Design review of the part built by this model. Coordinates are the model's own, in mm. Face numbers are marked on the shaded views. Coordinates: 2 decimals unless noted, no trailing zeros. Write each loop counter-clockwise with the first axis right and the second up, starting at its lowest first coordinate (ties: lowest second). Pieces come first, ordered by that corner, then holes. Notation, with made-up numbers: (-38, 41) -> (-29, 41) arc R30 ccw to (-29, 80) -> close; hole circle Ø8 at (78.25, 76). An arc over 180 degrees is marked (long way). Return JSON: item names as keys, results as strings. Group by question number.
from build123d import *

# Parameters (mm, degrees)
F1_DEPTH = 25.4


# Not quite as in the source:
# - ends of sketch curves that miss each other by under 0.0002 mm in the source are joined


with BuildPart() as f1:
    # F0 (on Front) → F1 (new body)
    with BuildSketch(Plane.XZ):
        with BuildLine():
            ThreePointArc((7.9345325801, 55.8050164826), (5.535399088, 50.3331676174), (0, 48.0845394904))
            ThreePointArc((0, 48.0845394904), (-5.53484385, 50.3326274112), (-7.9344900677, 55.8034677281))
            ThreePointArc((-7.9344900677, 55.8034677281), (-20.6052011609, 52.4624086595), (-32.1621766165, 46.2861708383))
            ThreePointArc((-32.1621766165, 46.2861708383), (-30.8592654267, 43.9476457313), (-30.4078463876, 41.3089911317))
            ThreePointArc((-30.4078463876, 41.3089911317), (-31.0665806395, 38.1430038554), (-32.9334464969, 35.5025080461))
            ThreePointArc((-32.9334464969, 35.5025080461), (-38.3527879746, 33.37149462), (-43.7681241803, 35.5126658077))
            ThreePointArc((-43.7681241803, 35.5126658077), (-51.6631141521, 22.5336801806), (-55.8055284532, 7.9177526246))
            ThreePointArc((-55.8055284532, 7.9177526246), (-50.5579583584, 5.4112130729), (-48.4275815127, 0))
            ThreePointArc((-48.4275815127, 0), (-50.5584477046, -5.4117381745), (-55.8069604277, -7.917853693))
            ThreePointArc((-55.8069604277, -7.917853693), (-51.6665413057, -22.5360169357), (-43.772503534, -35.5174627239))
            ThreePointArc((-43.772503534, -35.5174627239), (-38.3573927277, -33.3769597298), (-32.9385406353, -35.5079735997))
            ThreePointArc((-32.9385406353, -35.5079735997), (-31.0716747779, -38.1484694089), (-30.412940526, -41.3144566852))
            ThreePointArc((-30.412940526, -41.3144566852), (-30.8645222652, -43.9535728332), (-32.1678845367, -46.2923987991))
            ThreePointArc((-32.1678845367, -46.2923987991), (-20.6005666804, -52.4744238707), (-7.9177489459, -55.8160418449))
            ThreePointArc((-7.9177489459, -55.8160418449), (0.0007699496, -48.4381469932), (7.917857362, -55.8175779229))
            ThreePointArc((7.917857362, -55.8175779229), (20.6543242596, -52.4575865986), (32.263311311, -46.2335565237))
            ThreePointArc((32.263311311, -46.2335565237), (31.0776824279, -40.9625014731), (33.540338967, -36.1536492228))
            ThreePointArc((33.540338967, -36.1536492228), (38.5262504819, -34.0340714863), (43.7106191867, -35.607044642))
            ThreePointArc((43.7106191867, -35.607044642), (51.6543788303, -22.5889167608), (55.8178964863, -7.917853693))
            ThreePointArc((55.8178964863, -7.917853693), (48.4385176038, -0.0007177684), (55.8164645119, 7.9177526246))
            ThreePointArc((55.8164645119, 7.9177526246), (51.6724507462, 22.537346487), (43.7740191713, 35.5188777315))
            ThreePointArc((43.7740191713, 35.5188777315), (38.4803716898, 33.3779972711), (33.1194704023, 35.3444179256))
            ThreePointArc((33.1194704023, 35.3444179256), (33.0283665185, 35.4254890622), (32.9385189369, 35.5079503192))
            ThreePointArc((32.9385189369, 35.5079503192), (30.4331832399, 40.7476116526), (32.166542765, 46.2907355552))
            ThreePointArc((32.166542765, 46.2907355552), (20.6072932493, 52.4658819521), (7.9345325801, 55.8050164826))
        make_face()
        with BuildLine():
            ThreePointArc((0, 38.1), (13.962710806, 35.4492976933), (25.9825875048, 27.8660213621))
            ThreePointArc((25.9825875048, 27.8660213621), (34.9475216227, 15.1899725896), (38.1109370587, -0.010193824))
            ThreePointArc((38.1109370587, -0.010193824), (15.1973926464, -34.9527404783), (-25.9825835021, -27.8660170726))
            ThreePointArc((-25.9825835021, -27.8660170726), (-38.1, 0), (-25.9825875048, 27.8660213621))
            ThreePointArc((-25.9825875048, 27.8660213621), (-13.962710806, 35.4492976933), (0, 38.1))
        make_face(mode=Mode.SUBTRACT)
        with BuildLine():
            ThreePointArc((-32.1621766165, 46.2861708383), (-20.6052011609, 52.4624086595), (-7.9344900677, 55.8034677281))
            ThreePointArc((-7.9344900677, 55.8034677281), (-5.6894120792, 61.5568833403), (0, 63.9595394904))
            Line((0, 63.9595394904), (0, 73.9440789808))
            ThreePointArc((0, 73.9440789808), (-27.1479472531, 68.9440014522), (-50.7331165271, 54.5999571944))
            Line((-50.7331165271, 54.5999571944), (-43.7572462783, 47.1154742172))
            ThreePointArc((-43.7572462783, 47.1154742172), (-37.7790864379, 49.2262669207), (-32.1621766165, 46.2861708383))
        make_face()
        with BuildLine():
            ThreePointArc((7.9375, 56.0220394904), (7.9367581103, 55.9135178434), (7.9345325801, 55.8050164826))
            ThreePointArc((7.9345325801, 55.8050164826), (20.6072932493, 52.4658819521), (32.166542765, 46.2907355552))
            ThreePointArc((32.166542765, 46.2907355552), (37.7835970754, 49.2316689925), (43.7623187183, 47.1209164903))
            Line((43.7623187183, 47.1209164903), (50.7331165271, 54.5999571944))
            ThreePointArc((50.7331165271, 54.5999571944), (27.1479472531, 68.9440014522), (0, 73.9440789808))
            Line((0, 73.9440789808), (0, 63.9595394904))
            ThreePointArc((0, 63.9595394904), (5.6126600757, 61.634699566), (7.9375, 56.0220394904))
        make_face()
        with BuildLine():
            ThreePointArc((-43.7681241803, 35.5126658077), (-46.2828428993, 41.3164327187), (-43.7572462783, 47.1154742172))
            Line((-43.7572462783, 47.1154742172), (-50.7331165271, 54.5999571944))
            ThreePointArc((-50.7331165271, 54.5999571944), (-31.1494504015, -71.7983666167), (76.2, -2.2559210192))
            ThreePointArc((76.2, -2.2559210192), (69.5922116943, 28.7821857449), (50.9148537664, 54.4372678657))
            Line((50.9148537664, 54.4372678657), (43.9381604406, 46.9519018008))
            ThreePointArc((43.9381604406, 46.9519018008), (45.6769666267, 44.3682185312), (46.2879188276, 41.3144334048))
            ThreePointArc((46.2879188276, 41.3144334048), (45.6323737155, 38.1557882425), (43.7740191713, 35.5188777315))
            ThreePointArc((43.7740191713, 35.5188777315), (51.6724507462, 22.537346487), (55.8164645119, 7.9177526246))
            ThreePointArc((55.8164645119, 7.9177526246), (61.7872306442, 5.8071231544), (64.3135175714, 0))
            ThreePointArc((64.3135175714, 0), (61.7877557458, -5.8066338081), (55.8178964863, -7.917853693))
            ThreePointArc((55.8178964863, -7.917853693), (51.6543788303, -22.5889167608), (43.7106191867, -35.607044642))
            ThreePointArc((43.7106191867, -35.607044642), (46.0506031098, -38.4080721744), (46.8897388577, -41.9601323083))
            ThreePointArc((46.8897388577, -41.9601323083), (46.2310046059, -45.1261195846), (44.3641387485, -47.7666153939))
            ThreePointArc((44.3641387485, -47.7666153939), (37.9546080225, -49.8346887381), (32.263311311, -46.2335565237))
            ThreePointArc((32.263311311, -46.2335565237), (20.6543242596, -52.4575865986), (7.917857362, -55.8175779229))
            ThreePointArc((7.917857362, -55.8175779229), (7.9325878205, -56.0964396499), (7.9375, -56.3756469558))
            ThreePointArc((7.9375, -56.3756469558), (-0.2799767777, -64.3082076555), (-7.9177489459, -55.8160418449))
            ThreePointArc((-7.9177489459, -55.8160418449), (-20.6005666804, -52.4744238707), (-32.1678845367, -46.2923987991))
            ThreePointArc((-32.1678845367, -46.2923987991), (-37.784668716, -49.2317673719), (-43.7623404168, -47.1209397708))
            ThreePointArc((-43.7623404168, -47.1209397708), (-46.2879374814, -41.3214088869), (-43.772503534, -35.5174627239))
            ThreePointArc((-43.772503534, -35.5174627239), (-51.6665413057, -22.5360169357), (-55.8069604277, -7.917853693))
            ThreePointArc((-55.8069604277, -7.917853693), (-64.3025814803, 0.0007177684), (-55.8055284532, 7.9177526246))
            ThreePointArc((-55.8055284532, 7.9177526246), (-51.6631141521, 22.5336801806), (-43.7681241803, 35.5126658077))
        make_face()
    extrude(amount=F1_DEPTH)


solid = f1.part
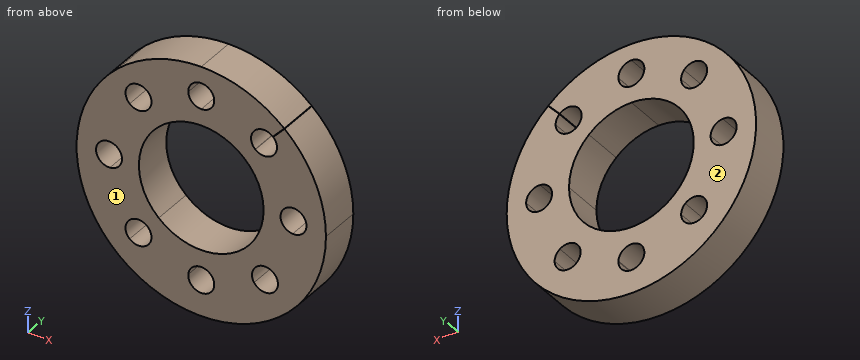
Q1. For P1, Ø1, axis at x = 7.5, y = -11.5, coming from the +Z side; P2, Ø5, axis at x = -29, z = 52, coming from the +Y side; P3, Ø1.5, axis at y = -5.5, z = 36, coming from the +X side; P4, Ø12, axis at x = 16.5, y = -11, coming from the -Z side, all flat-tipped, find the tip position at first contact; note any pin that passes through.
Q2. We need section A-A on x = -22.5. Write out the cut boundary in (y, z), plus the area to 3 significant figures.
Q3. We need section C-C on y = -9.25. State how many separate pieces and enclosed holes the cut face has, plus the area to 3 significant figures.
Q4. The part is to be moulded in two halves that separate along Y. For the marked faces 1 and 2, say which applies: +Y half, -Y half, draft (parallel to the pull), parting line (faces both ways), or undercut.
Q5. Wall thickness on L1, parallel to Z at x = -0.5, y = -7; L2, parallel to Z at x = -45, y = -19; L3, parallel to X at y = -19.5, z = 53: over which ranges is each line inside the solid? List them lowest first.
Q6. We need section B-B on x = 41. Write out the cut boundary in (y, z).
Q7. We need section D-D on x = -5.5. Write out the cut boundary in (y, z), plus the area to 3 significant figures.
Findings below:
{
 "1": {"P1": "stops at z = 73.62", "P2": "stops at y = 0", "P3": "stops at x = 66.33", "P4": "stops at z = -77.73"},
 "2": {"outline": "(-25.4, -75.06) -> (0, -75.06) -> (0, -30.75) -> (-25.4, -30.75) -> close; (-25.4, 30.75) -> (0, 30.75) -> (0, 70.55) -> (-25.4, 70.55) -> close", "area": "2,140 mm^2"},
 "3": {"separate pieces": "1", "enclosed holes": "8", "area": "12,100 mm^2"},
 "4": {"face 1": "-Y half", "face 2": "+Y half"},
 "5": {"L1": "z = -78.45 to -64.3, -48.45 to -38.11, 38.1 to 48.1, 63.94 to 73.94", "L2": "z = -63.75 to -45.65, -36.98 to 36.98, 45.64 to 59.24", "L3": "x = -52.47 to -7.34, 7.34 to 49.24, 49.58 to 52.47"},
 "6": {"outline": "(-25.4, -66.49) -> (0, -66.49) -> (0, -49.63) -> (-25.4, -49.63) -> close; (-25.4, -34.29) -> (0, -34.29) -> (0, 33.83) -> (-25.4, 33.83) -> close; (-25.4, 48.8) -> (0, 48.8) -> (0, 61.97) -> (-25.4, 61.97) -> close"},
 "7": {"outline": "(-25.4, -78.26) -> (0, -78.26) -> (0, -62.1) -> (-25.4, -62.1) -> close; (-25.4, -50.65) -> (0, -50.65) -> (0, -37.71) -> (-25.4, -37.71) -> close; (-25.4, 37.7) -> (0, 37.7) -> (0, 50.3) -> (-25.4, 50.3) -> close; (-25.4, 61.75) -> (0, 61.75) -> (0, 73.75) -> (-25.4, 73.75) -> close", "area": "1,360 mm^2"}
}
